from build123d import *

# Parameters (mm, degrees)
SKETCH1_R                = 10
BOSS_EXTRUDE1_DEPTH      = 6.35
SKETCH5_W                = 20
SKETCH5_H                = 30
BOSS_EXTRUDE2_DEPTH      = 6.35
SKETCH7_W                = 6.35
SKETCH7_H                = 30
BOSS_EXTRUDE3_DEPTH      = 120
BOSS_EXTRUDE3_DEPTH_BACK = 6.35
SKETCH8_R                = 9.75
CUT_EXTRUDE2_DEPTH       = 33.7
SKETCH2_R                = 4.7625
CUT_EXTRUDE1_DEPTH       = 7.35
FILLET2_R                = 10
SKETCH11_W               = 32.7
SKETCH11_H               = 35.8
BOSS_EXTRUDE5_DEPTH      = 6.35


with BuildPart() as part:
    # Sketch1 → Boss-Extrude1 (new body)
    with BuildSketch(Plane(origin=(0, 0, 0), x_dir=(1, 0, 0), z_dir=(0, 1, 0))):
        Circle(SKETCH1_R)
    extrude(amount=BOSS_EXTRUDE1_DEPTH)

    # Sketch5 → Boss-Extrude2 (add)
    with BuildSketch(Plane(origin=(0, 6.35, 0), x_dir=(1, 0, 0), z_dir=(0, 1, 0))):
        Rectangle(SKETCH5_W, SKETCH5_H)
    extrude(amount=-BOSS_EXTRUDE2_DEPTH)

    # Sketch7 → Boss-Extrude3 (add, two sides)
    with BuildSketch(Plane(origin=(0, 6.35, 0), x_dir=(1, 0, 0), z_dir=(0, 1, 0))) as boss_extrude3_sk:
        with Locations((-13.175, 0)):
            Rectangle(SKETCH7_W, SKETCH7_H)
        with Locations((13.175, 0)):
            Rectangle(SKETCH7_W, SKETCH7_H)
    extrude(amount=BOSS_EXTRUDE3_DEPTH)
    extrude(boss_extrude3_sk.sketch, amount=-BOSS_EXTRUDE3_DEPTH_BACK)

    # Sketch8 → Cut-Extrude2 (cut, through all)
    with BuildSketch(Plane.ZY.offset(16.35)):
        with Locations((0, 100.95)):
            Circle(SKETCH8_R)
    extrude(amount=-CUT_EXTRUDE2_DEPTH, mode=Mode.SUBTRACT)

    # Sketch2 → Cut-Extrude1 (cut, through all)
    with BuildSketch(Plane(origin=(0, 6.35, 0), x_dir=(1, 0, 0), z_dir=(0, 1, 0))):
        Circle(SKETCH2_R)
    extrude(amount=-CUT_EXTRUDE1_DEPTH, mode=Mode.SUBTRACT)

    # Fillet2
    fillet2_edges = [part.edges().sort_by_distance(p)[0] for p in [
        (13.175, 126.35, -15),
        (13.175, 126.35, 15),
        (-13.175, 126.35, 15),
        (-13.175, 126.35, -15),
    ]]
    fillet(fillet2_edges, radius=FILLET2_R)

    # Sketch11 → Boss-Extrude5 (add)
    with BuildSketch(Plane.XZ):
        with Locations((0, -32.9)):
            Rectangle(SKETCH11_W, SKETCH11_H)
    extrude(amount=-BOSS_EXTRUDE5_DEPTH)


solid = part.part
CAD build for the part. Positions are in the model's coordinates, mm. A direction names the side the tool comes from. Round coordinates to 2 decimals unless told otherwise and drop trailing zeros. Loops run counter-clockwise (first coordinate to the right, second up) from the corner with the lowest first, then second, coordinate; pieces in that order, holes last. Notation, with made-up numbers: (-1, 77.25) - (41, 77.25) arc R12 cw to (41, 81.25) - close; hole circle Ø8 at (41, 46.5). An arc over 180 degrees is marked (long way). Put each result on its own line as item: value.
1. Slice it at D-D on x = 14.5. List the corners of the cut face in (y, z), and give its area (3 significant figures).
Geometry check:
outline: (0, -50.8) - (6.35, -50.8) - (6.35, -15) - (116.35, -15) arc R10 ccw to (126.35, -5) - (126.35, 5) arc R10 ccw to (116.35, 15) - (0, 15) - close; hole circle Ø19.5 at (100.95, 0)
area: 3,680 mm²
2. Slice it at A-A on x = 0. List the corners of the cut face in (y, z).
Geometry check:
outline: (0, -50.8) - (6.35, -50.8) - (6.35, -4.76) - (0, -4.76) - close; (0, 4.76) - (6.35, 4.76) - (6.35, 15) - (0, 15) - close
3. Slice it at C-C on z = 0. List the corners of the cut face in (x, y).
Geometry check:
outline: (-16.35, 0) - (-4.76, 0) - (-4.76, 6.35) - (-10, 6.35) - (-10, 91.2) - (-16.35, 91.2) - close; (-16.35, 110.7) - (-10, 110.7) - (-10, 126.35) - (-16.35, 126.35) - close; (4.76, 0) - (16.35, 0) - (16.35, 91.2) - (10, 91.2) - (10, 6.35) - (4.76, 6.35) - close; (10, 110.7) - (16.35, 110.7) - (16.35, 126.35) - (10, 126.35) - close
4. 3-axis set-ups, long thin cutter, end or side, ignore diameter. For faces 1 (the flat face through (13, 62, -15)), 2 (the flat face through (-10, 66, 0)), 3 (the flat face through (0, 3, -50.8)): which of +Z, -Z, +X, -X, +Y, -Y reach the whole face in a straight line?
Geometry check:
face 1: -Z, +X, -X, +Y
face 2: +Z, -Z, +Y
face 3: -Z, +X, -X, +Y, -Y
5. Slice it at B-B on y = 96. List the corners of the cut face in (x, z), and give its area (3 significant figures).
Geometry check:
outline: (-16.35, -15) - (-10, -15) - (-10, -8.4) - (-16.35, -8.4) - close; (-16.35, 8.4) - (-10, 8.4) - (-10, 15) - (-16.35, 15) - close; (10, -15) - (16.35, -15) - (16.35, -8.4) - (10, -8.4) - close; (10, 8.4) - (16.35, 8.4) - (16.35, 15) - (10, 15) - close
area: 168 mm²
6. Two-plate mould, pull along X, no slides. Class faces 4 (the cylindrical face through (13.13, 91.43, -2.11)), 5 (the flat face through (0, 6.35, -25)), 6 (the flat face through (16.35, 48, -4)), 7 (the cylindrical face through (-3.78, 3.22, 2.9)): released by +X, released by -X, zero draft, split by the parting line, or undercut.
Geometry check:
face 4: zero draft
face 5: undercut
face 6: released by +X
face 7: undercut
7. Wall check: line 1 (X direction, y = 40, z = -14); line 2 (X direction, y = 2, z = 0); line 3 (Z direction, x = 0, y = 2). Give the ranges that are in metal, low to high.
Geometry check:
line 1: -16.35 to -10, 10 to 16.35
line 2: -16.35 to -4.76, 4.76 to 16.35
line 3: -50.8 to -4.76, 4.76 to 15
8. Pin check, flat tips, straight feed: P1, Ø1.5, axis at x = 10.5, z = -6.5, coming from the +Y side; P2, Ø7, axis at x = -13, y = 35.5, coming from the -Z side; P3, Ø4, axis at x = 12.5, z = -29, coming from the +Y side. Stop position of each tip, or through.
Geometry check:
P1: y = 126.32
P2: z = -15
P3: y = 6.35
